The listing builds one solid part. Answer for the finished solid, in the listing's coordinates (mm). A direction names the side the tool comes from. Coordinates: 2 decimals unless noted, no trailing zeros. Write each loop counter-clockwise with the first axis right and the second up, starting at its lowest first coordinate (ties: lowest second). Pieces come first, ordered by that corner, then holes. Notation, with made-up numbers: M 19,60 L 63,60 A12 ccw 63,65 Z; hole C 28.5,58.25 d3. An arc over 180 degrees is marked long. Answer as CSV lines item,"result".
```python
from build123d import *

# Parameters (mm, degrees)
SKETCH1_W               = 130
SKETCH1_H               = 24
BOSS_EXTRUDE1_DEPTH     = 5
CUT_EXTRUDE1_DEPTH      = 133.291345144
CUT_EXTRUDE1_DEPTH_BACK = 133.291345144
SKETCH2_R               = 6.5
SKETCH3_R               = 12
BOSS_EXTRUDE3_DEPTH     = 10
SKETCH4_R               = 6.5
CUT_EXTRUDE2_DEPTH      = 5
CUT_EXTRUDE3_DEPTH      = 133.574507353
CUT_EXTRUDE3_DEPTH_BACK = 133.574507353
BOSS_EXTRUDE4_DEPTH     = 2
SKETCH7_W               = 20
SKETCH7_H               = 5
BOSS_EXTRUDE5_DEPTH     = 205
SKETCH8_W               = 20
SKETCH8_H               = 5
BOSS_EXTRUDE6_DEPTH     = 28
SKETCH9_W               = 20
SKETCH9_H               = 5
BOSS_EXTRUDE7_DEPTH     = 18
SKETCH10_W              = 5
SKETCH10_H              = 10
BOSS_EXTRUDE8_DEPTH     = 25
SKETCH11_W              = 5
SKETCH11_H              = 10
BOSS_EXTRUDE9_DEPTH     = 25
SKETCH12_R              = 1.5
CUT_EXTRUDE4_DEPTH      = 188.59530911
THICKEN1_T2             = 3
THICKEN2_START          = 22
THICKEN2_DEPTH          = 3
THICKEN3_START          = 5
THICKEN3_DEPTH          = 3
THICKEN4_START          = 105
THICKEN4_DEPTH          = 3
CUT_EXTRUDE5_REACH      = 258.984
SKETCH14_R              = 1.5


# Read off the part's stored shape, not the designer's step: Thicken2, Thicken3, Thicken4
with BuildPart() as part:
    # Sketch1 → Boss-Extrude1 (new body)
    with BuildSketch(Plane.XY):
        with Locations((65, 12)):
            Rectangle(SKETCH1_W, SKETCH1_H)
    extrude(amount=BOSS_EXTRUDE1_DEPTH)

    # Sketch2 → Cut-Extrude1 (cut, two sides: drawn at the far end of the back side and taken through both)
    with BuildSketch(Plane(origin=(0, 0, 0), x_dir=(-1, 0, 0), z_dir=(0, 0, -1)).offset(-CUT_EXTRUDE1_DEPTH_BACK)):
        with Locations((-15, 12)):
            Circle(SKETCH2_R)
        with Locations((-115, 12)):
            Circle(SKETCH2_R)
    extrude(amount=CUT_EXTRUDE1_DEPTH + CUT_EXTRUDE1_DEPTH_BACK, mode=Mode.SUBTRACT)

    # Sketch3 → Boss-Extrude3 (add)
    with BuildSketch(Plane.XY.offset(5)):
        with Locations(Location((15, 12, 0), (0, 0, 270))):
            Circle(SKETCH3_R)
        with Locations(Location((115, 12, 0), (0, 0, 270))):
            Circle(SKETCH3_R)
    extrude(amount=BOSS_EXTRUDE3_DEPTH)

    # Sketch4 → Cut-Extrude2 (cut)
    with BuildSketch(Plane(origin=(0, 0, 5), x_dir=(-1, 0, 0), z_dir=(0, 0, -1))):
        with Locations((-15, 12)):
            Circle(SKETCH4_R)
        with Locations((-115, 12)):
            Circle(SKETCH4_R)
    extrude(amount=-CUT_EXTRUDE2_DEPTH, mode=Mode.SUBTRACT)

    # Sketch5 → Cut-Extrude3 (cut, two sides: drawn at the far end of the back side and taken through both)
    with BuildSketch(Plane.XY.offset(5).offset(-CUT_EXTRUDE3_DEPTH_BACK)):
        with BuildLine():
            Line((3, 24), (0, 24))
            Line((0, 24), (0, 0))
            Line((0, 0), (15, 0))
            ThreePointArc((15, 0), (6.514718626, 3.514718626), (3, 12))
            Line((3, 12), (3, 24))
        make_face()
        with BuildLine():
            Line((115, 0), (130, 0))
            Line((130, 0), (130, 24))
            Line((130, 24), (127, 24))
            Line((127, 24), (127, 12))
            ThreePointArc((127, 12), (123.485281374, 3.514718626), (115, 0))
        make_face()
    extrude(amount=CUT_EXTRUDE3_DEPTH + CUT_EXTRUDE3_DEPTH_BACK, mode=Mode.SUBTRACT)

    # Sketch6 → Boss-Extrude4 (add)
    with BuildSketch(Plane(origin=(0, 24, 0), x_dir=(1, 0, 0), z_dir=(0, 1, 0))):
        Polygon((127, 0), (3, 0), (3, -5), (15, -5), (115, -5), (127, -5), align=None)
    extrude(amount=BOSS_EXTRUDE4_DEPTH)

    # Sketch7 → Boss-Extrude5 (add)
    with BuildSketch(Plane(origin=(0, 0, 0), x_dir=(-1, 0, 0), z_dir=(0, 0, -1))):
        with Locations((-115, 23.5)):
            Rectangle(SKETCH7_W, SKETCH7_H)
        with Locations((-15, 23.5)):
            Rectangle(SKETCH7_W, SKETCH7_H)
    extrude(amount=BOSS_EXTRUDE5_DEPTH)

    # Sketch8 → Boss-Extrude6 (add)
    with BuildSketch(Plane(origin=(0, 26, 0), x_dir=(1, 0, 0), z_dir=(0, 1, 0))):
        with Locations((115, 111.5)):
            Rectangle(SKETCH8_W, SKETCH8_H)
        with Locations((15, 111.5)):
            Rectangle(SKETCH8_W, SKETCH8_H)
    extrude(amount=BOSS_EXTRUDE6_DEPTH)

    # Sketch9 → Boss-Extrude7 (add)
    with BuildSketch(Plane(origin=(0, 26, 0), x_dir=(1, 0, 0), z_dir=(0, 1, 0))):
        with Locations((115, 202.5)):
            Rectangle(SKETCH9_W, SKETCH9_H)
        with Locations((15, 202.5)):
            Rectangle(SKETCH9_W, SKETCH9_H)
    extrude(amount=BOSS_EXTRUDE7_DEPTH)

    # Sketch10 → Boss-Extrude8 (add)
    with BuildSketch(Plane.ZY.offset(-105)):
        with Locations((-111.5, 49)):
            Rectangle(SKETCH10_W, SKETCH10_H)
    extrude(amount=-BOSS_EXTRUDE8_DEPTH)

    # Sketch11 → Boss-Extrude9 (add)
    with BuildSketch(Plane(origin=(25, 0, 0), x_dir=(0, 0, -1), z_dir=(1, 0, 0))):
        with Locations((111.5, 49)):
            Rectangle(SKETCH11_W, SKETCH11_H)
    extrude(amount=-BOSS_EXTRUDE9_DEPTH)

    # Sketch12 → Cut-Extrude4 (cut, through all)
    with BuildSketch(Plane.XY.offset(-109)):
        with Locations((124.874085346, 48.801077027)):
            Circle(SKETCH12_R)
        with Locations((114.374085346, 48.801077027)):
            Circle(SKETCH12_R)
        with Locations((15.624085346, 48.801077027)):
            Circle(SKETCH12_R)
        with Locations((5.124085346, 48.801077027)):
            Circle(SKETCH12_R)
    extrude(amount=-CUT_EXTRUDE4_DEPTH, mode=Mode.SUBTRACT)

    # Sketch13 → Surface-Plane1: a flat surface bounded by the sketch
    with BuildSketch(Plane(origin=(125, 0, 0), x_dir=(0, 0, -1), z_dir=(1, 0, 0)), mode=Mode.PRIVATE) as surface_plane1_1_region:
        Polygon((109, 44), (109, 26), (89, 26), align=None)
    surface_plane1_1 = surface_plane1_1_region.sketch.faces()[0]
    add(Solid.thicken(surface_plane1_1, -THICKEN1_T2))

    # Thicken2 outline → Thicken2 (add)
    with BuildSketch(Plane.YZ.offset(THICKEN2_START)):
        Polygon((44, -109), (26, -89), (26, -109), align=None)
    extrude(amount=THICKEN2_DEPTH)

    # Thicken3 outline → Thicken3 (add)
    with BuildSketch(Plane.YZ.offset(THICKEN3_START)):
        Polygon((44, -109), (26, -89), (26, -109), align=None)
    extrude(amount=THICKEN3_DEPTH)

    # Thicken4 outline → Thicken4 (add)
    with BuildSketch(Plane.YZ.offset(THICKEN4_START)):
        Polygon((44, -109), (26, -89), (26, -109), align=None)
    extrude(amount=THICKEN4_DEPTH)

    # Sketch14 → Cut-Extrude5 (cut, up to next)
    with BuildSketch(Plane.XY.offset(-200), mode=Mode.PRIVATE) as cut_extrude5_sk1:
        with Locations((109.5, 36)):
            Circle(SKETCH14_R)
    cut_extrude5_tool1 = extrude(cut_extrude5_sk1.sketch, amount=-CUT_EXTRUDE5_REACH, mode=Mode.PRIVATE) & part.part
    # Sketch14 → Cut-Extrude5 (cut, up to next)
    with BuildSketch(Plane.XY.offset(-200), mode=Mode.PRIVATE) as cut_extrude5_sk2:
        with Locations((120.5, 36)):
            Circle(SKETCH14_R)
    cut_extrude5_tool2 = extrude(cut_extrude5_sk2.sketch, amount=-CUT_EXTRUDE5_REACH, mode=Mode.PRIVATE) & part.part
    # Sketch14 → Cut-Extrude5 (cut, up to next)
    with BuildSketch(Plane.XY.offset(-200), mode=Mode.PRIVATE) as cut_extrude5_sk3:
        with Locations((9.5, 36)):
            Circle(SKETCH14_R)
    cut_extrude5_tool3 = extrude(cut_extrude5_sk3.sketch, amount=-CUT_EXTRUDE5_REACH, mode=Mode.PRIVATE) & part.part
    # Sketch14 → Cut-Extrude5 (cut, up to next)
    with BuildSketch(Plane.XY.offset(-200), mode=Mode.PRIVATE) as cut_extrude5_sk4:
        with Locations((20.5, 36)):
            Circle(SKETCH14_R)
    cut_extrude5_tool4 = extrude(cut_extrude5_sk4.sketch, amount=-CUT_EXTRUDE5_REACH, mode=Mode.PRIVATE) & part.part
    add(cut_extrude5_tool1.solids().sort_by_distance((109.5, 36, -200))[0], mode=Mode.SUBTRACT)
    add(cut_extrude5_tool2.solids().sort_by_distance((120.5, 36, -200))[0], mode=Mode.SUBTRACT)
    add(cut_extrude5_tool3.solids().sort_by_distance((9.5, 36, -200))[0], mode=Mode.SUBTRACT)
    add(cut_extrude5_tool4.solids().sort_by_distance((20.5, 36, -200))[0], mode=Mode.SUBTRACT)


solid = part.part
```
Q1. Find section C-C (y = 8). Give the vertices of the cut face in (x, z).
Output:
outline,"M 3.69,0 L 9.88,0 L 9.88,10 L 20.12,10 L 20.12,0 L 109.88,0 L 109.88,10 L 120.12,10 L 120.12,0 L 126.31,0 L 126.31,15 L 103.69,15 L 103.69,5 L 26.31,5 L 26.31,15 L 3.69,15 Z"
Q2. Straight lines are drawn through the part: line 1 (Y direction, x = 115, z = 7); line 2 (Z direction, x = 10.5, y = 33); line 3 (X direction, y = 25, z = -40.5). For each, find the intervals that lie inside material, in ascending order.
Output:
line 1,"0 to 5.5, 18.5 to 24"
line 2,"-205 to -200, -114 to -109"
line 3,"5 to 25, 105 to 125"
Q3. Find section B-B (x = 67.5). Give the vertices of the cut face in (y, z), and give its area (3 significant figures).
Output:
outline,"M 0,0 L 26,0 L 26,5 L 0,5 Z"
area,"130 mm2"
Q4. Find section A-A (z = -146). Give the vertices of the cut face in (x, y), and give its area (3 significant figures).
Output:
outline,"M 5,21 L 25,21 L 25,26 L 5,26 Z; M 105,21 L 125,21 L 125,26 L 105,26 Z"
area,"200 mm2"
Q5. The mould has two halves that part along Y. Classify faces 5 (the cylindrical face through (121.494, 12.286, 5.07)), 6 (the flat face through (15, 21, -101)), 7 (the flat face through (125, 26, -111)): pulls with the +Y half, pulls with the -Y half, needs draft (parallel to the pull), parting line crosses it, or undercut.
Output:
face 5,"undercut"
face 6,"pulls with the -Y half"
face 7,"needs draft"
Q6. Flat-ended cylindrical pins translate along their axes: pin 1 Ø2 at (x, z) = (23.5, -87.5) entering from -Y; pin 2 Ø2.5 at (x, y) = (120.5, 36) entering from -Z; pin 3 Ø5.5 at (y, z) = (31, -101.5) entering from +X. Find the tip coordinate at first contact, or state that the pin passes through.
Output:
pin 1,"y = 21"
pin 2,"z = -114"
pin 3,"x = 125"
Q7. For faces 1 (the cylindrical face through (10.404, 0.915, 9.062)), 2 (the flat face through (15, 40, -114)), 3 (the flat face through (22, 31, -103)), 4 (the flat face through (127, 44, -112)), determine the directions among +Z, -Z, +X, -X, +Y, -Y from which every point of the face is accessible in a straight line to the end or side of a thin tool.
Output:
face 1,"+Z"
face 2,"+X, -X, +Y"
face 3,"+Z, +Y"
face 4,"+Z, -Z, +X, -Y"
